CAD build for the part. Positions are in the model's coordinates, mm. Face numbers are marked on the shaded views. A direction names the side the tool comes from. Give positions to 0.01 mm unless a question says otherwise; leave off trailing zeros. Loops run counter-clockwise (first coordinate to the right, second up) from the corner with the lowest first, then second, coordinate; pieces in that order, holes last. Notation, with made-up numbers: M -5,-10 L 19,-10 A18 ccw 19,25 Z; hole C 69,19.5 d10. An arc over 180 degrees is marked long. One line per question, with ' | ' between items.
```python
from build123d import *

# Parameters (mm, degrees)
BOSS_EXTRUDE1_DEPTH = 6.35


with BuildPart() as part:
    # Sketch1 → Boss-Extrude1 (new body)
    with BuildSketch(Plane.XY):
        with BuildLine():
            Line((-5.08, 17.78), (5.08, 17.78))
            Line((5.08, 17.78), (5.08, 11.639742265))
            ThreePointArc((5.08, 11.639742265), (0, -12.7), (-5.08, 11.639742265))
            Line((-5.08, 11.639742265), (-5.08, 17.78))
        make_face()
        Polygon((7.332348419, 0), (3.666174209, 6.35), (-3.666174209, 6.35), (-7.332348419, 0), (-3.666174209, -6.35), (3.666174209, -6.35), align=None, mode=Mode.SUBTRACT)
    extrude(amount=BOSS_EXTRUDE1_DEPTH)


solid = part.part
```
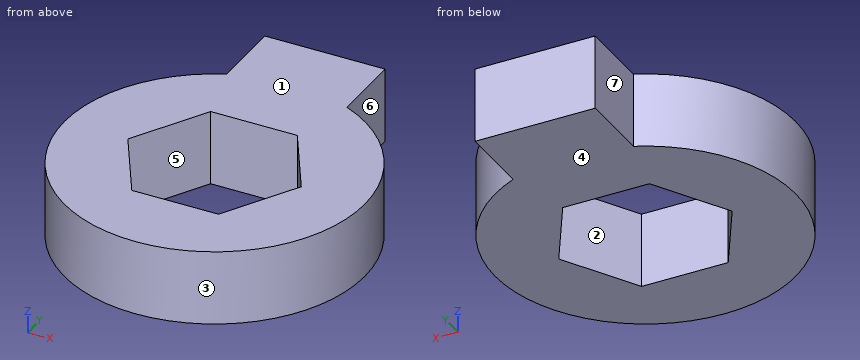
Item 1: Saw through at A-A on x = 0. Give the cut face in (y, z), and give its area (3 significant figures).
Conclusion:
outline: M -12.7,0 L -6.35,0 L -6.35,6.35 L -12.7,6.35 Z; M 6.35,0 L 17.78,0 L 17.78,6.35 L 6.35,6.35 Z | area: 113 mm²
Item 2: Drill centre lines: line 1 along X through (y, z) = (1, 6) (3 decimals); line 2 along Y through (x, z) = (-6.75, 3.25); line 3 along X through (y, z) = (13, 3). Where is each one in solid material? Low to high. Write a range as [from, to].
Conclusion:
line 1: [-12.661, -6.755], [6.755, 12.661] | line 2: [-10.76, -1.01], [1.01, 10.76] | line 3: [-5.08, 5.08]
Item 3: 3-axis set-ups, long thin cutter, end or side, ignore diameter. For the marked faces 4, 5, 6 and 7: which of +Z, -Z, +X, -X, +Y, -Y reach the whole face in a straight line?
Conclusion:
face 4: -Z, +X, -X, +Y, -Y | face 5: +Z, -Z | face 6: +Z, -Z, +X, +Y | face 7: +Z, -Z, -X, +Y
Item 4: Mould opens along Y. For the marked faces 1, 2 and 3 say: pulls with the +Y half, pulls with the -Y half, needs draft (parallel to the pull), parting line crosses it, or undercut.
Conclusion:
face 1: needs draft | face 2: undercut | face 3: parting line crosses it
Item 5: Saw through at D-D on x = -10.75. Give the cut face in (y, z).
Conclusion:
outline: M -6.76,0 L 6.76,0 L 6.76,6.35 L -6.76,6.35 Z
Item 6: Drop a flat-ended pin along its axis: P1, Ø1.8, axis at y = 13.5, z = 4, coming from the +X side. Give the stop position or say it passes through.
Conclusion:
P1: x = 5.08
Item 7: Saw through at B-B on y = -6. Give the cut face in (x, z), and give its area (3 significant figures).
Conclusion:
outline: M -11.19,0 L -3.87,0 L -3.87,6.35 L -11.19,6.35 Z; M 3.87,0 L 11.19,0 L 11.19,6.35 L 3.87,6.35 Z | area: 93.0 mm²
Item 8: Saw through at C-C on z = 3.5. Give the cut face in (x, y).
Conclusion:
outline: M -5.08,11.64 A12.7 ccw long 5.08,11.64 L 5.08,17.78 L -5.08,17.78 Z; hole M -7.33,0 L -3.67,-6.35 L 3.67,-6.35 L 7.33,0 L 3.67,6.35 L -3.67,6.35 Z
